Autodesk Inventor part; units mm, degrees
ref_plane "YZ Plane" through (0, 0, 0) normal (1, 0, 0) x (0, 1, 0)
ref_plane "XZ Plane" through (0, 0, 0) normal (0, 1, 0) x (-1, 0, 0)
ref_plane "XY Plane" through (0, 0, 0) normal (0, 0, 1) x (1, 0, 0)
sketch "Sketch15" plane through (0, 0, 0) normal (0, 0, 1) x (1, 0, 0)
  line L0 (0, 0) -> (0, 2.5)
  line L1 (0.2887, 3) -> (2.25, 3)
  line L2 (3, 4.4) -> (3, 4.4)
  line L3 (2.25, 1.5) -> (6.25, 1.5)
  line L4 (6.25, 0) -> (0, 0)
  line L5 (0.2887, 3) -> (0, 2.5)
  line L6 (2.25, 1.5) -> (2.25, 3)
  line L7 (6.25, 1.5) -> (6.25, 0)
  dimension "d83" = 30
  dimension "d84" = 1.5
  dimension "d86" = 0.5
  dimension "d87" = 3
  dimension "d116" = 2.25
  dimension "d117" = 4
revolve "Revolution1" add sketch "Sketch15" angle 360 about axis through (6.25, 0, 0) along (-1, 0, 0)
sketch "Sketch16" plane through (0, 0, 0) normal (-1, 0, 0) x (0, 0, 1)
  circle A0 centre (0, 0) radius 2.5
  line L0 (1.5, 2.5981) -> (3, 0)
  line L1 (3, 0) -> (1.5, -2.5981)
  line L2 (1.5, -2.5981) -> (-1.5, -2.5981)
  line L3 (-1.5, -2.5981) -> (-3, 0)
  line L4 (-3, 0) -> (-1.5, 2.5981)
  line L5 (-1.5, 2.5981) -> (1.5, 2.5981)
  circle A1 centre (0, 0) radius 5.2707
  dimension "d128" = 3
extrude "Extrusion15" cut sketch "Sketch16" against normal blind 5 contours A1
chamfer "Chamfer5" distance 0.2 angle 45 1 edges at (6.25, -1.5, 0)
thread "Thread7"
sketch "Sketch19" plane through (2.25, -2.5981, 1.5) normal (1, 0, 0) x (0, 0, -1)
  circle A0 centre (1.5, 2.5981) radius 1.5
  circle A1 centre (1.5, 2.5981) radius 4
  dimension "d131" = 8
extrude "Extrusion18" add sketch "Sketch19" along normal blind 0.5
sketch "Boceto20" plane through (0, 0, 0) normal (-1, 0, 0) x (0, 0, 1)
  circle A0 centre (0, 0) radius 1.3
properties part number "Bolt3W" material "Acero, alta resistencia, aleación baja"
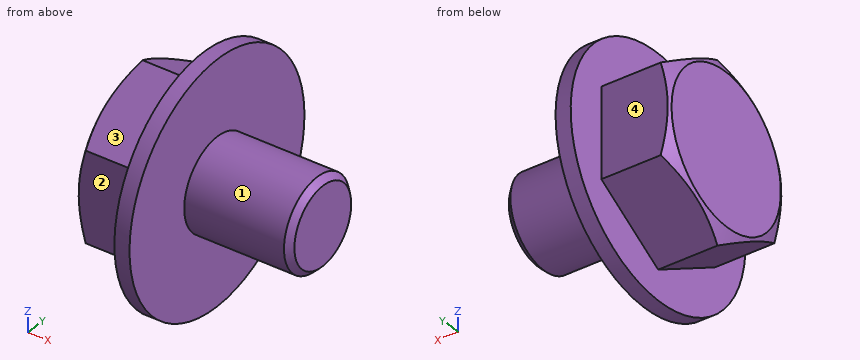
Could you check a few things on this model? Use its own coordinates, in mm. Face numbers are marked on the shaded views. A direction names the side the tool comes from. Coordinates: 2 decimals unless noted, no trailing zeros. Write each loop counter-clockwise with the first axis right and the second up, starting at its lowest first coordinate (ties: lowest second). Pieces come first, ordered by that corner, then holes. Notation, with made-up numbers: (59, -16.75) - (89, -16.75) arc R16 ccw to (89, -7.75) - close; hole circle Ø9 at (84.25, 3). An arc over 180 degrees is marked (long way). Use a Markdown table: item, result.
Q1. I'm going to push flat-ended pins straight in: pin 1 Ø0.7 at (x, z) = (0.5, 0.5) entering from +Y; pin 2 Ø1.8 at (x, z) = (1, 0) entering from -Y. Where does each tip first touch, or does it pass through?
Geometry check:
| item | result |
|---|---|
| pin 1 | stops at y = 2.6 |
| pin 2 | stops at y = -2.6 |
Q2. Please list where these lines run through material, in increasing order: L1, parallel to X at y = 2, z = 3; L2, parallel to Z at x = 3.75, y = -0.75; L3, parallel to Y at x = 4, z = 0.
Geometry check:
| item | result |
|---|---|
| L1 | x = 2.25 to 2.75 |
| L2 | z = -1.3 to 1.3 |
| L3 | y = -1.5 to 1.5 |
Q3. Which directions (+Z, -Z, +X, -X, +Y, -Y) give clear straight access to the entire face, cutting with the end or side of a thin tool? Please do the marked faces 1, 2, 3 and 4.
Geometry check:
| item | result |
|---|---|
| face 1 | +X |
| face 2 | +Z, -Z, -X, -Y |
| face 3 | +Z, -X, -Y |
| face 4 | +Z, -Z, -X, +Y |
Q4. Imagine slicing it at C-C (x = 2.5). List the corners of the cut face in (y, z) for me.
Geometry check:
| item | result |
|---|---|
| outline | circle Ø8 at (0, 0) |
Q5. Imagine slicing it at A-A (z = 0). List the corners of the cut face in (x, y) for me.
Geometry check:
| item | result |
|---|---|
| outline | (0, -2.5) - (0.06, -2.6) - (2.25, -2.6) - (2.25, -4) - (2.75, -4) - (2.75, -1.5) - (6.05, -1.5) - (6.25, -1.3) - (6.25, 1.3) - (6.05, 1.5) - (2.75, 1.5) - (2.75, 4) - (2.25, 4) - (2.25, 2.6) - (0.06, 2.6) - (0, 2.5) - close |
Q6. Imagine slicing it at D-D (y = 3.5). List the corners of the cut face in (x, z) for me.
Geometry check:
| item | result |
|---|---|
| outline | (2.25, -1.94) - (2.75, -1.94) - (2.75, 1.94) - (2.25, 1.94) - close |
